Part model, mm, in its own coordinate system. Face numbers are marked on the shaded views. A direction names the side the tool comes from. Round coordinates to 2 decimals unless told otherwise and drop trailing zeros. Write each loop counter-clockwise with the first axis right and the second up, starting at its lowest first coordinate (ties: lowest second). Pieces come first, ordered by that corner, then holes. Notation, with made-up numbers: (39, 47.25) -> (63, 47.25) arc R25 ccw to (63, 67.25) -> close; hole circle Ø11 at (25, -34). An arc over 180 degrees is marked (long way). Use CSV: the item, a comma, the result in double quotes. Start each with the question number.
(1) Drop flat-ended pins along their axis: pin 1 (3 mm diameter, centred on y = 2.5, z = -32.5, fed in from +X); pin 2 (1.1 mm diameter, centred on x = -9.5, z = -68, fed in from +Y); pin 3 (10 mm diameter, centred on x = -19.5, z = -69, fed in from -Y); pin 4 (2 mm diameter, centred on y = 31.5, z = -176, fed in from +X). Give the stop position or say it passes through.
(2) Saw through at C-C (z = -153). Give the cut face in (x, y).
(3) Probe line 1 (Z direction, x = -5.5, y = 11); line 2 (Y direction, x = -9.35, z = -4.5); line 3 (X direction, y = 19.5, z = -70). List the from-to ranges inside material, lowest first. Write a range as [from, to].
(4) Two-plate mould, pull along Z, no slides. Class the marked faces 3, 4 and 5: released by +Z, released by -Z, zero draft, split by the parting line, or undercut.
(5) Saw through at B-B (x = -52.5). Give the cut face in (y, z), plus the area to 3 significant figures.
(6) Saw through at A-A (y = 15.5). Give the cut face in (x, z).
(7) Which spindle directions (+Z, -Z, +X, -X, +Y, -Y) get a long thin tool onto all of the face, cutting with end or side? Do the marked faces 1 and 2. Say none if no direction does.
```python
from build123d import *
from OCP.BRepFilletAPI import BRepFilletAPI_MakeChamfer

# Parameters (mm, degrees)
SKETCH1_W           = 68.5
SKETCH1_H           = 64.5
BOSS_EXTRUDE3_DEPTH = 21
SKETCH3_W           = 61.5
SKETCH3_H           = 61
CUT_EXTRUDE1_DEPTH  = 15
SKETCH5_W           = 68.5
SKETCH5_H           = 6
BOSS_EXTRUDE4_DEPTH = 105
SKETCH10_W          = 10
SKETCH10_H          = 29
BOSS_EXTRUDE5_DEPTH = 5.5
SKETCH9_W           = 3.5
SKETCH9_H           = 20
CUT_EXTRUDE2_DEPTH  = 20.5
SKETCH11_W          = 6
SKETCH11_H          = 20
CUT_EXTRUDE3_DEPTH  = 5.5
CHAMFER2_SIZE       = 5.5
CHAMFER2_SIZE_2     = 5
CHAMFER3_SIZE       = 2
SKETCH12_W          = 34.25
SKETCH12_H          = 169.5
CUT_EXTRUDE4_DEPTH  = 50
SKETCH15_R          = 1.5
CUT_EXTRUDE5_DEPTH  = 50
SKETCH19_W          = 34.25
SKETCH19_H          = 6
BOSS_EXTRUDE6_DEPTH = 11
SKETCH26_W          = 12
SKETCH26_H          = 9
BOSS_EXTRUDE7_DEPTH = 30
SKETCH20_R          = 3.75
CUT_EXTRUDE9_DEPTH  = 188.119113134
SKETCH21_W          = 3
SKETCH21_H          = 2.806985986
CUT_EXTRUDE10_DEPTH = 188.119113134
SKETCH18_R          = 1.5
CUT_EXTRUDE8_DEPTH  = 135
SKETCH24_R          = 4
CUT_EXTRUDE13_DEPTH = 196.377839071
SKETCH25_W          = 3
SKETCH25_H          = 3.218590937
CUT_EXTRUDE14_DEPTH = 196.377839071
SKETCH33_R          = 1.5
CUT_EXTRUDE17_DEPTH = 9.74
SKETCH34_R          = 3.75
CUT_EXTRUDE18_DEPTH = 196.377839071
SKETCH39_W          = 3
SKETCH39_H          = 4.471117771
CUT_EXTRUDE22_DEPTH = 196.377839071
CUT_EXTRUDE23_DEPTH = 15
SKETCH41_W          = 4.5
SKETCH41_H          = 9
CUT_EXTRUDE24_DEPTH = 9
SKETCH42_R          = 1.25
CUT_EXTRUDE25_DEPTH = 197.388645293
SKETCH43_W          = 12
SKETCH43_H          = 9
BOSS_EXTRUDE8_DEPTH = 4
SKETCH44_W          = 4.5
SKETCH44_H          = 9
CUT_EXTRUDE26_DEPTH = 9
SKETCH45_R          = 1.25
CUT_EXTRUDE27_DEPTH = 198.16110164


with BuildPart() as part:
    # Sketch1 → Boss-Extrude3 (new body)
    with BuildSketch(Plane(origin=(0, 0, 0), x_dir=(1, 0, 0), z_dir=(0, 1, 0))):
        with Locations((-34.25, 32.25)):
            Rectangle(SKETCH1_W, SKETCH1_H)
    extrude(amount=BOSS_EXTRUDE3_DEPTH)

    # Sketch3 → Cut-Extrude1 (cut)
    with BuildSketch(Plane(origin=(0, 21, 0), x_dir=(1, 0, 0), z_dir=(0, 1, 0))):
        with Locations((-34.25, 34)):
            Rectangle(SKETCH3_W, SKETCH3_H)
    extrude(amount=-CUT_EXTRUDE1_DEPTH, mode=Mode.SUBTRACT)

    # Sketch5 → Boss-Extrude4 (add)
    with BuildSketch(Plane(origin=(0, 0, -64.5), x_dir=(-1, 0, 0), z_dir=(0, 0, -1))):
        with Locations((34.25, 3)):
            Rectangle(SKETCH5_W, SKETCH5_H)
    extrude(amount=BOSS_EXTRUDE4_DEPTH)

    # Sketch10 → Boss-Extrude5 (add)
    with BuildSketch(Plane.XZ):
        with Locations((-5, -30)):
            Rectangle(SKETCH10_W, SKETCH10_H)
    extrude(amount=BOSS_EXTRUDE5_DEPTH)

    # Sketch9 → Cut-Extrude2 (cut)
    with BuildSketch(Plane(origin=(0, 21, 0), x_dir=(1, 0, 0), z_dir=(0, 1, 0))):
        with Locations((-1.75, 28)):
            Rectangle(SKETCH9_W, SKETCH9_H)
    extrude(amount=-CUT_EXTRUDE2_DEPTH, mode=Mode.SUBTRACT)

    # Sketch11 → Cut-Extrude3 (cut)
    with BuildSketch(Plane(origin=(0, 6, 0), x_dir=(1, 0, 0), z_dir=(0, 1, 0))):
        with Locations((-6.5, 28)):
            Rectangle(SKETCH11_W, SKETCH11_H)
    extrude(amount=-CUT_EXTRUDE3_DEPTH, mode=Mode.SUBTRACT)

    # Chamfer2
    chamfer2_edges_1 = [part.edges().sort_by_distance(p)[0] for p in [
        (-5, -5.5, -44.5),
    ]]
    chamfer2_side_1 = [part.faces().sort_by_distance(p)[0] for p in [
        (-5, -5.4, -44.5),
    ]]
    chamfer2_edges_2 = [part.edges().sort_by_distance(p)[0] for p in [
        (-5, -5.5, -15.5),
    ]]
    chamfer2_side_2 = [part.faces().sort_by_distance(p)[0] for p in [
        (-5, -5.5, -15.6),
    ]]
    chamfer2 = BRepFilletAPI_MakeChamfer(part.part.solid().wrapped)
    for e in chamfer2_edges_1:
        chamfer2.Add(CHAMFER2_SIZE - 0.0001, CHAMFER2_SIZE_2 - 0.0001, e.wrapped, chamfer2_side_1[0].wrapped)
    for e in chamfer2_edges_2:
        chamfer2.Add(CHAMFER2_SIZE_2 - 0.0001, CHAMFER2_SIZE - 0.0001, e.wrapped, chamfer2_side_2[0].wrapped)
    add(Compound.cast(chamfer2.Shape()), mode=Mode.REPLACE)  # a hair under: the kernel refuses the full size

    # Chamfer3
    chamfer3_edges = [part.edges().sort_by_distance(p)[0] for p in [
        (-4.75, 0.5, -38),
        (-4.75, 0.5, -18),
    ]]
    chamfer(chamfer3_edges, length=CHAMFER3_SIZE)

    # Sketch12 → Cut-Extrude4 (cut)
    with BuildSketch(Plane(origin=(0, 21, 0), x_dir=(1, 0, 0), z_dir=(0, 1, 0))):
        with Locations((-51.375, 84.75)):
            Rectangle(SKETCH12_W, SKETCH12_H)
    extrude(amount=-CUT_EXTRUDE4_DEPTH, mode=Mode.SUBTRACT)

    # Sketch15 → Cut-Extrude5 (cut)
    with BuildSketch(Plane(origin=(0, 0.5, 0), x_dir=(1, 0, 0), z_dir=(0, 1, 0))):
        with Locations(Location((-4, 31.75713966, 0), (0, 0, 270))):
            Circle(SKETCH15_R)
    extrude(amount=-CUT_EXTRUDE5_DEPTH, mode=Mode.SUBTRACT)

    # Sketch19 → Boss-Extrude6 (add)
    with BuildSketch(Plane(origin=(0, 0, -169.5), x_dir=(-1, 0, 0), z_dir=(0, 0, -1))):
        with Locations((17.125, 3)):
            Rectangle(SKETCH19_W, SKETCH19_H)
    extrude(amount=BOSS_EXTRUDE6_DEPTH)

    # Sketch26 → Boss-Extrude7 (add)
    with BuildSketch(Plane(origin=(0, 6, 0), x_dir=(1, 0, 0), z_dir=(0, 1, 0))):
        with Locations((-6, 69)):
            Rectangle(SKETCH26_W, SKETCH26_H)
        with Locations((-6, 4.5)):
            Rectangle(SKETCH26_W, SKETCH26_H)
        with Locations((-6, 176)):
            Rectangle(SKETCH26_W, SKETCH26_H)
    extrude(amount=BOSS_EXTRUDE7_DEPTH)

    # Sketch20 → Cut-Extrude9 (cut, through all)
    with BuildSketch(Plane(origin=(0, 0.5, 0), x_dir=(1, 0, 0), z_dir=(0, 1, 0))):
        with Locations(Location((-4.5, 25.778009288, 0), (0, 0, 270))):
            Circle(SKETCH20_R)
    extrude(amount=-CUT_EXTRUDE9_DEPTH, mode=Mode.SUBTRACT)

    # Sketch21 → Cut-Extrude10 (cut, through all)
    with BuildSketch(Plane(origin=(0, 0.5, 0), x_dir=(1, 0, 0), z_dir=(0, 1, 0))):
        with Locations((-4, 30.353646667)):
            Rectangle(SKETCH21_W, SKETCH21_H)
    extrude(amount=-CUT_EXTRUDE10_DEPTH, mode=Mode.SUBTRACT)

    # Mirror5: part across plane


with BuildPart() as part_1:
    add(part.part)
    add(part.part.mirror(Plane(origin=(-34.25, 0, 0), x_dir=(0, 0, 1), z_dir=(1, 0, 0))))

    # Sketch18 → Cut-Extrude8 (cut)
    with BuildSketch(Plane(origin=(0, 6, 0), x_dir=(1, 0, 0), z_dir=(0, 1, 0))):
        with Locations(Location((-12, 167.25713966, 0), (0, 0, 270))):
            Circle(SKETCH18_R)
    extrude(amount=-CUT_EXTRUDE8_DEPTH, mode=Mode.SUBTRACT)

    # Sketch24 → Cut-Extrude13 (cut, through all)
    with BuildSketch(Plane(origin=(0, 6, 0), x_dir=(1, 0, 0), z_dir=(0, 1, 0))):
        with Locations(Location((-12, 161.25713966, 0), (0, 0, 270))):
            Circle(SKETCH24_R)
    extrude(amount=-CUT_EXTRUDE13_DEPTH, mode=Mode.SUBTRACT)

    # Sketch25 → Cut-Extrude14 (cut, through all)
    with BuildSketch(Plane(origin=(0, 6, 0), x_dir=(1, 0, 0), z_dir=(0, 1, 0))):
        with Locations((-12, 165.647844192)):
            Rectangle(SKETCH25_W, SKETCH25_H)
    extrude(amount=-CUT_EXTRUDE14_DEPTH, mode=Mode.SUBTRACT)

    # Sketch33 → Cut-Extrude17 (cut)
    with BuildSketch(Plane(origin=(0, 6, 0), x_dir=(1, 0, 0), z_dir=(0, 1, 0))):
        with Locations(Location((-64.5, 167.25713966, 0), (0, 0, 270))):
            Circle(SKETCH33_R)
        with Locations((-64.5, 31.75713966)):
            Circle(SKETCH33_R)
        with Locations((-12, 167.25713966)):
            Circle(SKETCH33_R)
    extrude(amount=-CUT_EXTRUDE17_DEPTH, mode=Mode.SUBTRACT)

    # Sketch34 → Cut-Extrude18 (cut, through all)
    with BuildSketch(Plane(origin=(0, 6, 0), x_dir=(1, 0, 0), z_dir=(0, 1, 0))):
        with Locations(Location((-64, 161.278009288, 0), (0, 0, 270))):
            Circle(SKETCH34_R)
    extrude(amount=-CUT_EXTRUDE18_DEPTH, mode=Mode.SUBTRACT)

    # Sketch39 → Cut-Extrude22 (cut, through all)
    with BuildSketch(Plane(origin=(0, 6, 0), x_dir=(1, 0, 0), z_dir=(0, 1, 0))):
        with Locations((-64.5, 165.021580775)):
            Rectangle(SKETCH39_W, SKETCH39_H)
    extrude(amount=-CUT_EXTRUDE22_DEPTH, mode=Mode.SUBTRACT)

    # Sketch40 → Cut-Extrude23 (cut)
    with BuildSketch(Plane(origin=(0, 21, 0), x_dir=(1, 0, 0), z_dir=(0, 1, 0))):
        Polygon((-68.5, 64.5), (-68.5, 9), (-56.5, 9), (-56.5, 0), (-12, 0), (-12, 9), (0, 9), (0, 64.5), align=None)
    extrude(amount=-CUT_EXTRUDE23_DEPTH, mode=Mode.SUBTRACT)

    # Sketch41 → Cut-Extrude24 (cut)
    with BuildSketch(Plane(origin=(0, 36, 0), x_dir=(1, 0, 0), z_dir=(0, 1, 0))):
        with Locations((-62.5, 69)):
            Rectangle(SKETCH41_W, SKETCH41_H)
        with Locations((-62.5, 176)):
            Rectangle(SKETCH41_W, SKETCH41_H)
        with Locations((-6, 69)):
            Rectangle(SKETCH41_W, SKETCH41_H)
        with Locations((-6, 176)):
            Rectangle(SKETCH41_W, SKETCH41_H)
    extrude(amount=-CUT_EXTRUDE24_DEPTH, mode=Mode.SUBTRACT)

    # Sketch42 → Cut-Extrude25 (cut, through all)
    with BuildSketch(Plane(origin=(0, 0, 0), x_dir=(0, 0, -1), z_dir=(1, 0, 0))):
        with Locations((69, 31.5)):
            Circle(SKETCH42_R)
        with Locations((176, 31.5)):
            Circle(SKETCH42_R)
    extrude(amount=-CUT_EXTRUDE25_DEPTH, mode=Mode.SUBTRACT)

    # Sketch43 → Boss-Extrude8 (add)
    with BuildSketch(Plane(origin=(0, 36, 0), x_dir=(1, 0, 0), z_dir=(0, 1, 0))):
        with Locations((-62.5, 4.5)):
            Rectangle(SKETCH43_W, SKETCH43_H)
        with Locations((-6, 4.5)):
            Rectangle(SKETCH43_W, SKETCH43_H)
    extrude(amount=BOSS_EXTRUDE8_DEPTH)

    # Sketch44 → Cut-Extrude26 (cut)
    with BuildSketch(Plane(origin=(0, 40, 0), x_dir=(1, 0, 0), z_dir=(0, 1, 0))):
        with Locations((-62.5, 4.5)):
            Rectangle(SKETCH44_W, SKETCH44_H)
        with Locations((-6, 4.5)):
            Rectangle(SKETCH44_W, SKETCH44_H)
    extrude(amount=-CUT_EXTRUDE26_DEPTH, mode=Mode.SUBTRACT)

    # Sketch45 → Cut-Extrude27 (cut, through all)
    with BuildSketch(Plane(origin=(0, 0, 0), x_dir=(0, 0, -1), z_dir=(1, 0, 0))):
        with Locations((4.5, 35.5)):
            Circle(SKETCH45_R)
    extrude(amount=-CUT_EXTRUDE27_DEPTH, mode=Mode.SUBTRACT)


solid = part_1.part
```
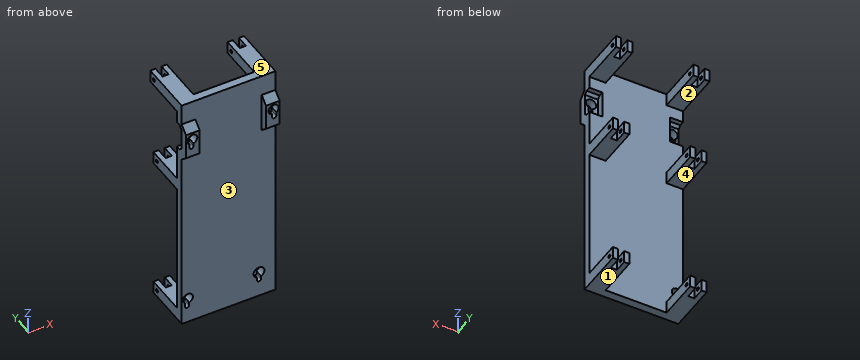
Answers:
1,pin 1,"stops at x = -9.5"
1,pin 2,"stops at y = 36"
1,pin 3,"stops at y = 0"
1,pin 4,"passes through"
2,outline,"(-68.5, 0) -> (0, 0) -> (0, 6) -> (-68.5, 6) -> close"
3,line 1,"z = [-180.5, -171.5], [-73.5, -64.5], [-9, 0]"
3,line 2,"y = [0, 34.25], [36.75, 40]"
3,line 3,"x = [-68.5, -56.5], [-12, 0]"
4,face 3,"zero draft"
4,face 4,"undercut"
4,face 5,"released by +Z"
5,outline,"(0, -180.5) -> (6, -180.5) -> (6, 0) -> (0, 0) -> close"
5,area,"1,080 mm²"
6,outline,"(-68.5, -180.5) -> (-56.5, -180.5) -> (-56.5, -171.5) -> (-68.5, -171.5) -> close; (-68.5, -73.5) -> (-56.5, -73.5) -> (-56.5, -64.5) -> (-68.5, -64.5) -> close; (-68.5, -9) -> (-56.5, -9) -> (-56.5, 0) -> (-68.5, 0) -> close; (-12, -180.5) -> (0, -180.5) -> (0, -171.5) -> (-12, -171.5) -> close; (-12, -73.5) -> (0, -73.5) -> (0, -64.5) -> (-12, -64.5) -> close; (-12, -9) -> (0, -9) -> (0, 0) -> (-12, 0) -> close"
7,face 1,"-Z, +X, -X, +Y, -Y"
7,face 2,"+X, -X, +Y"
